Verification items for the finished model (mm, model axes). Face numbers are marked on the shaded views. A direction names the side the tool comes from. Round coordinates to 2 decimals unless told otherwise and drop trailing zeros. Write each loop counter-clockwise with the first axis right and the second up, starting at its lowest first coordinate (ties: lowest second). Pieces come first, ordered by that corner, then holes. Notation, with made-up numbers: (86.25, 4) -> (144.25, 4) arc R30 ccw to (144.25, 28) -> close; hole circle Ø2 at (49.5, -10.75). An arc over 180 degrees is marked (long way). Answer as a JSON object with one key per item and string values. Group by question number.
(1) Sectioned sample at A-A on y = 0. Record the cut outline in (x, z).
(2) Sectioned sample at B-B on z = 2.5. Record the cut outline in (x, y).
(3) Gauge pin test, flat ends, axial feed: pin 1 Ø2 at (x, z) = (2.5, -1) entering from +Y (3 decimals); pin 2 Ø9.5 at (x, y) = (14.72, 8.5) entering from +Z; pin 3 Ø9.5 at (x, y) = (0, 17) entering from -Z; pin 4 Ø3.5 at (x, y) = (-14.72, -8.5) entering from +Z. Record the tip position at first contact, or that the pin passes through.
(4) Scan lines: L1, parallel to Y at x = 0, z = -2.75; L2, parallel to Y at x = 0, z = -13; L3, parallel to Y at x = 0, z = 8.25. Record each from-to range of solid material in increasing order. Write a range as from..to.
(5) Sectioned sample at C-C on x = 0. Count the separate pieces of the cut face and the enclosed holes in it, and give its area (3 significant figures).
(6) Set-up check for the marked faces 1, 2, 3, 4 and 5: record each of +Z, -Z, +X, -X, +Y, -Y from which the full face is reachable in a straight line by a thin tool's end or side.
(7) Draft check along X on the marked faces 6, 7 and 8. Enter one of: released by +X, released by -X, zero draft, split by the parting line, or undercut.
```python
from build123d import *

# Parameters (mm, degrees)
SKETCH1_R                = 50
SKETCH1_R_2              = 10
BOSS_EXTRUDE1_DEPTH      = 15
SKETCH2_R                = 32.5
CUT_EXTRUDE2_DEPTH       = 10
SKETCH3_R                = 3
CUT_EXTRUDE8_DEPTH       = 10
CIRPATTERN1_COUNT        = 6
BOSS_EXTRUDE3_DEPTH      = 2
BOSS_EXTRUDE3_DEPTH_BACK = 7
SKETCH4_R                = 11
SKETCH4_R_2              = 10


with BuildPart() as part:
    # Sketch1 → Boss-Extrude1 (new, symmetric)
    with BuildSketch(Plane.XY):
        Circle(SKETCH1_R)
        Circle(SKETCH1_R_2, mode=Mode.SUBTRACT)
    extrude(amount=BOSS_EXTRUDE1_DEPTH, both=True)

    # Sketch2 → Cut-Extrude2 (cut)
    with BuildSketch(Plane.XY.offset(15)):
        Circle(SKETCH2_R)
    cut_extrude2 = extrude(amount=-CUT_EXTRUDE2_DEPTH, mode=Mode.SUBTRACT)

    # Mirror2: Cut-Extrude2 across plane
    add(cut_extrude2.mirror(Plane.XY), mode=Mode.SUBTRACT)

    # Sketch3 → Cut-Extrude8 (cut)
    with BuildSketch(Plane.XY.offset(5)):
        with Locations((0, 17)):
            Circle(SKETCH3_R)
    cut_extrude8 = extrude(amount=-CUT_EXTRUDE8_DEPTH, mode=Mode.SUBTRACT)

    # CirPattern1: Cut-Extrude8 ×6 about axis
    cirpattern1_axis = Axis((0, 0, 0), (0, 0, 1))
    for i in range(1, CIRPATTERN1_COUNT):
        add(cut_extrude8.rotate(cirpattern1_axis, i * 360 / CIRPATTERN1_COUNT), mode=Mode.SUBTRACT)

    # Sketch4 → Boss-Extrude3 (add, two sides: drawn at the far end of the back side and taken through both)
    with BuildSketch(Plane.XY.offset(5).offset(-BOSS_EXTRUDE3_DEPTH_BACK)):
        Circle(SKETCH4_R)
        with Locations(Location((0, 0, 0), (0, 0, 180))):
            Circle(SKETCH4_R_2, mode=Mode.SUBTRACT)
    extrude(amount=BOSS_EXTRUDE3_DEPTH + BOSS_EXTRUDE3_DEPTH_BACK)

    # Sketch5 → Cut-Revolve2 (revolve, cut)
    with BuildSketch(Plane(origin=(0, 0, 0), x_dir=(1, 0, 0), z_dir=(0, 1, 0))):
        Polygon((50, 12), (45, 9.113248654), (45, -9.113248654), (50, -12), align=None)
    revolve(axis=Axis((0, 0, 0), (0, 0, -1)), mode=Mode.SUBTRACT)


solid = part.part
```
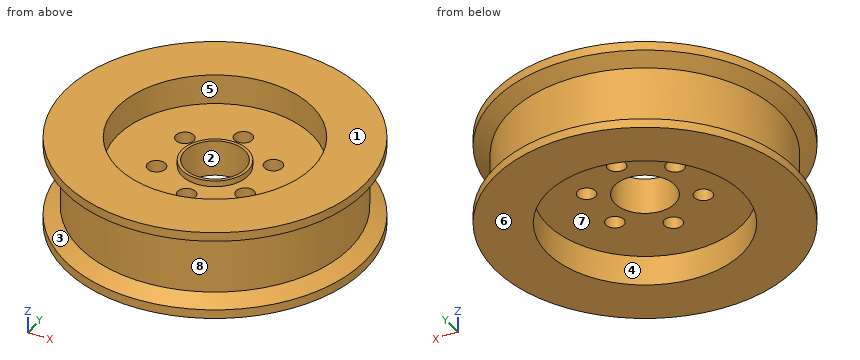
Computed values:
{
 "1": {"outline": "(-50, -15) -> (-32.5, -15) -> (-32.5, -5) -> (-10, -5) -> (-10, 7) -> (-11, 7) -> (-11, 5) -> (-32.5, 5) -> (-32.5, 15) -> (-50, 15) -> (-50, 12) -> (-45, 9.11) -> (-45, -9.11) -> (-50, -12) -> close; (10, -5) -> (32.5, -5) -> (32.5, -15) -> (50, -15) -> (50, -12) -> (45, -9.11) -> (45, 9.11) -> (50, 12) -> (50, 15) -> (32.5, 15) -> (32.5, 5) -> (11, 5) -> (11, 7) -> (10, 7) -> close"},
 "2": {"outline": "circle Ø90 at (0, 0); hole circle Ø6 at (-14.72, -8.5); hole circle Ø6 at (-14.72, 8.5); hole circle Ø20 at (0, 0); hole circle Ø6 at (0, -17); hole circle Ø6 at (0, 17); hole circle Ø6 at (14.72, -8.5); hole circle Ø6 at (14.72, 8.5)"},
 "3": {"pin 1": "y = 44.975", "pin 2": "z = 5", "pin 3": "z = -5", "pin 4": "through"},
 "4": {"L1": "-45..-20, -14..-10, 10..14, 20..45", "L2": "-50..-32.5, 32.5..50", "L3": "-45..-32.5, 32.5..45"},
 "5": {"separate pieces": "4", "enclosed holes": "0", "area": "1,170 mm2"},
 "6": {"face 1": "+Z, +X, -X, +Y, -Y", "face 2": "+Z, -Z", "face 3": "none", "face 4": "-Z", "face 5": "+Z"},
 "7": {"face 6": "zero draft", "face 7": "undercut", "face 8": "split by the parting line"}
}
